Read the model definition and answer for the solid it produces. Units are mm, in the model's axes. A direction names the side the tool comes from. Give positions to 0.01 mm unless a question says otherwise; leave off trailing zeros. Loops run counter-clockwise (first coordinate to the right, second up) from the corner with the lowest first, then second, coordinate; pieces in that order, holes last. Notation, with made-up numbers: (57, -17) -> (74, -17) arc R24 ccw to (74, 3) -> close; hole circle Ø11 at (64.25, 57.5). An arc over 180 degrees is marked (long way). Write each question's results on one line, items separated by ' | '. Start each with the question number.
Item 1: Each of these flat-tipped pins is pushed along its axis until it touches: P1, Ø17.5, axis at x = -4, z = -9.5, coming from the -Y side; P2, Ø19.5, axis at x = 8, y = -32.5, coming from the +Z side; P3, Ø5, axis at x = -17.5, y = -10.5, coming from the -Z side. Where does it stop, or does it pass through?
Item 2: Determine the mould class of faces 5 (the cylindrical face through (-25.11, -0.285, -26.199)), 6 (the cylindrical face through (25.11, -0.285, 26.199)), 7 (the cylindrical face through (-48.92, -12.59, -28.85)), 8 (the flat face through (1, 0, 0)) for opening direction Z: +Z half, -Z half, draft (parallel to the pull), parting line (faces both ways), or undercut.
Item 3: Section C-C on x = 6 is taken. Write down the section's boundary in (y, z).
Item 4: Section A-A on x = -43.5 is taken. Write down the section's boundary in (y, z), and give its area (3 significant figures).
Item 5: Section B-B on z = 5.5 is taken. Write down the section's boundary in (x, y).
Item 6: Find the intervals of material crossed by line 1 (X direction, y = -10, z = -8); line 2 (Z direction, x = 14.5, y = -32); line 3 (Y direction, x = 44, z = -8), in increasing order.
Item 7: Which of the six approach directions +Z, -Z, +X, -X, +Y, -Y give full straight-line access (tool end or side, diameter ignored) to faces 1 (the cylindrical face through (25.236, -0.285, -26.288)), 2 (the flat face through (0, -25, -22.979)), 3 (the flat face through (-24.937, -19.07, 26.446)), 4 (the flat face through (-1, -4, 0))?
```python
from build123d import *

# Parameters (mm, degrees)
SKETCH1_R           = 3.286752884
BOSS_EXTRUDE2_DEPTH = 50
FILLET1_R           = 2
FILLET2_R           = 1
CUT_EXTRUDE1_DEPTH  = 70
SKETCH3_W           = 0.91909433
SKETCH3_H           = 44.79975758
CUT_EXTRUDE3_DEPTH  = 46


with BuildPart() as part:
    # Sketch1 → Boss-Extrude2 (new body)
    with BuildSketch(Plane(origin=(0, 0, 0), x_dir=(1, 0, 0), z_dir=(0, 1, 0))):
        Polygon((-50, -30), (-50, 30), (-30, 30), (-20, 22.979280262), (20, 22.979280262), (30, 30), (50, 30), (50, -30), (30, -30), (20, -22.979280262), (-20, -22.979280262), (-30, -30), align=None)
        with Locations(Location((-44.920732924, 24.848491151, 0), (0, 0, 270))):
            Circle(SKETCH1_R, mode=Mode.SUBTRACT)
        with Locations(Location((-44.920732924, -24.848491151, 0), (0, 0, 90))):
            Circle(SKETCH1_R, mode=Mode.SUBTRACT)
        with Locations(Location((44.920732924, -24.848491151, 0), (0, 0, 270))):
            Circle(SKETCH1_R, mode=Mode.SUBTRACT)
        with Locations(Location((44.920732924, 24.848491151, 0), (0, 0, 90))):
            Circle(SKETCH1_R, mode=Mode.SUBTRACT)
    extrude(amount=-BOSS_EXTRUDE2_DEPTH)

    # Fillet1
    fillet1_edges = [part.edges().sort_by_distance(p)[0] for p in [
        (-30, -25, -30),
        (-20, -25, -22.979280262),
        (20, -25, -22.979280262),
        (30, -25, -30),
        (50, -25, -30),
        (50, -25, 30),
        (30, -25, 30),
        (20, -25, 22.979280262),
        (-20, -25, 22.979280262),
        (-30, -25, 30),
        (-50, -25, 30),
        (-50, -25, -30),
    ]]
    fillet(fillet1_edges, radius=FILLET1_R)

    # Fillet2
    fillet2_edges = [part.edges().sort_by_distance(p)[0] for p in [
        (-39.315986035, 0, -30),
        (-50, 0, 0),
        (-39.315986035, 0, 30),
        (-25, 0, 26.489640131),
        (0, 0, 22.979280262),
        (25, 0, 26.489640131),
        (39.315986035, 0, 30),
        (50, 0, 0),
        (39.315986035, 0, -30),
        (25, 0, -26.489640131),
        (0, 0, -22.979280262),
        (-25, 0, -26.489640131),
        (-49.414213562, 0, 29.414213562),
        (-30.029368482, 0, 29.907057659),
        (30.029368482, 0, 29.907057659),
        (49.414213562, 0, 29.414213562),
        (49.414213562, 0, -29.414213562),
        (30.029368482, 0, -29.907057659),
        (-30.029368482, 0, -29.907057659),
        (-49.414213562, 0, -29.414213562),
        (-19.970631518, 0, -23.072222603),
        (19.970631518, 0, -23.072222603),
        (19.970631518, 0, 23.072222603),
        (-19.970631518, 0, 23.072222603),
    ]]
    fillet(fillet2_edges, radius=FILLET2_R)

    # Sketch2 → Cut-Extrude1 (cut)
    with BuildSketch(Plane.XY.offset(30)):
        Polygon((-48, -50), (-30.631972071, -50), (-30.631972071, -31.387227089), (-48, -20.62903259), align=None)
        with BuildLine():
            Line((-30.631972071, -50), (-0.459547165, -50))
            ThreePointArc((-0.459547165, -50), (-4.852357389, -48.649438504), (-8.06664868, -45.364757467))
            Line((-8.06664868, -45.364757467), (-30.631972071, -31.387227089))
            Line((-30.631972071, -31.387227089), (-30.631972071, -50))
        make_face()
        with BuildLine():
            ThreePointArc((8.06664868, -45.364757467), (4.852357389, -48.649438504), (0.459547165, -50))
            Line((0.459547165, -50), (50, -50))
            Line((50, -50), (50, -19.390182152))
            Line((50, -19.390182152), (8.06664868, -45.364757467))
        make_face()
        Polygon((-50, -50), (-48, -50), (-48, -20.62903259), (-50, -19.390182152), align=None)
        with BuildLine():
            ThreePointArc((3.5, -40.686020198), (2.474873734, -38.211146463), (0, -37.186020198))
            Line((0, -37.186020198), (0, -44.186020198))
            ThreePointArc((0, -44.186020198), (2.474873734, -43.160893932), (3.5, -40.686020198))
        make_face()
        with BuildLine():
            Line((0, -44.186020198), (0, -37.186020198))
            ThreePointArc((0, -37.186020198), (-3.5, -40.686020198), (0, -44.186020198))
        make_face()
    extrude(amount=-CUT_EXTRUDE1_DEPTH, mode=Mode.SUBTRACT)

    # Sketch3 → Cut-Extrude3 (cut)
    with BuildSketch(Plane.XZ.offset(50)):
        with BuildLine():
            Line((-0.459547165, -22.39987879), (-0.459547165, 22.39987879))
            Line((-0.459547165, 22.39987879), (-20.353496243, 22.39987879))
            Line((-20.353496243, 22.39987879), (-30.352042537, 29.450884636))
            Line((-30.352042537, 29.450884636), (-47.491946123, 29.450884636))
            ThreePointArc((-47.491946123, 29.450884636), (-48.906159685, 28.865098198), (-49.491946123, 27.450884636))
            Line((-49.491946123, 27.450884636), (-49.491946123, 0.606224364))
            Line((-49.491946123, 0.606224364), (-49.491946123, 0))
            Line((-49.491946123, 0), (-49.491946123, -0.606224364))
            Line((-49.491946123, -0.606224364), (-49.491946123, -27.450884636))
            ThreePointArc((-49.491946123, -27.450884636), (-48.906159685, -28.865098198), (-47.491946123, -29.450884636))
            Line((-47.491946123, -29.450884636), (-30.352042537, -29.450884636))
            Line((-30.352042537, -29.450884636), (-20.353496243, -22.39987879))
            Line((-20.353496243, -22.39987879), (-0.459547165, -22.39987879))
        make_face()
        Rectangle(SKETCH3_W, SKETCH3_H)
        with BuildLine():
            Line((47.491946123, 29.450884636), (30.352042537, 29.450884636))
            Line((30.352042537, 29.450884636), (20.353496243, 22.39987879))
            Line((20.353496243, 22.39987879), (0.459547165, 22.39987879))
            Line((0.459547165, 22.39987879), (0.459547165, -22.39987879))
            Line((0.459547165, -22.39987879), (20.353496243, -22.39987879))
            Line((20.353496243, -22.39987879), (30.352042537, -29.450884636))
            Line((30.352042537, -29.450884636), (47.491946123, -29.450884636))
            ThreePointArc((47.491946123, -29.450884636), (48.906159685, -28.865098198), (49.491946123, -27.450884636))
            Line((49.491946123, -27.450884636), (49.491946123, -0.606224364))
            Line((49.491946123, -0.606224364), (49.491946123, 0.606224364))
            Line((49.491946123, 0.606224364), (49.491946123, 27.450884636))
            ThreePointArc((49.491946123, 27.450884636), (48.906159685, 28.865098198), (47.491946123, 29.450884636))
        make_face()
    extrude(amount=-CUT_EXTRUDE3_DEPTH, mode=Mode.SUBTRACT)


solid = part.part
```
Findings:
1) P1: y = -4 | P2: z = 22.98 | P3: z = -23.08
2) face 5: -Z half | face 6: +Z half | face 7: undercut | face 8: draft
3) outline: (-47.82, -22.98) -> (-1, -22.98) arc R1 ccw to (0, -21.98) -> (0, 21.98) arc R1 ccw to (-1, 22.98) -> (-47.82, 22.98) -> (-47.82, 22.4) -> (-4, 22.4) -> (-4, -22.4) -> (-47.82, -22.4) -> close
4) outline: (-23.42, -30) -> (-1, -30) arc R1 ccw to (0, -29) -> (0, -27.81) -> (-4, -27.81) -> (-4, -29.45) -> (-23.42, -29.45) -> close; (-23.42, 29.45) -> (-4, 29.45) -> (-4, 27.81) -> (0, 27.81) -> (0, 29) arc R1 ccw to (-1, 30) -> (-23.42, 30) -> close; (-4, -21.88) -> (0, -21.88) -> (0, 21.88) -> (-4, 21.88) -> close | area: 213 mm2
5) outline: (-50, -19.39) -> (-49.49, -19.7) -> (-49.49, -4) -> (49.49, -4) -> (49.49, -19.7) -> (50, -19.39) -> (50, -1) arc R1 ccw to (49, 0) -> (-49, 0) arc R1 ccw to (-50, -1) -> close
6) line 1: -50 to -49.49, 49.49 to 50 | line 2: -22.98 to -22.4, 22.4 to 22.98 | line 3: -4 to 0
7) face 1: -Z, +Y | face 2: -Z, +Y, -Y | face 3: +Z, +Y, -Y | face 4: -Y
